Here's how the part is built. I have some questions about the finished solid (model axes, mm). A direction names the side the tool comes from. Round coordinates to 2 decimals unless told otherwise and drop trailing zeros. Write each loop counter-clockwise with the first axis right and the second up, starting at its lowest first coordinate (ties: lowest second). Pieces come first, ordered by that corner, then holes. Notation, with made-up numbers: (44.5, 47) - (101.5, 47) arc R28 ccw to (101.5, 73) - close; hole circle Ø7 at (37.5, 43). An arc over 180 degrees is marked (long way). Write item = value, one per line. Start each with the question number.
Item 1: If we section it at B-B (x = -73.5): Please give me the cut outline in (y, z).
Item 2: Which directions (+Z, -Z, +X, -X, +Y, -Y) give clear straight access to the entire face, cutting with the end or side of a thin tool? Please do faces 4 (the face through (6.37, 0.67, -105.56)), 5 (the face through (6, 54, -106.35)), 6 (the face through (2, 0, -1)).
Item 3: If we section it at A-A (y = 34): Please give me the cut outline in (x, z), and give its area (3 significant figures).
Item 4: If I drill on line 1 along Z through (x, y) = (10.5, 49.5); line 2 along Y through (x, z) = (47, -3.5); line 3 along X through (y, z) = (25, -90.5), over which ranges is the centre line in solid material (lowest first)? Write a range as [from, to].
Item 5: Thinking about a two-plate mould opening in Z: for faces 1 (the face through (-173.4, 54, -1)), 2 (the face through (1.58, 0.67, 105.56)), 3 (the face through (2, 54, 106.35)), which applies, pulls with the +Z half, pulls with the -Z half, needs draft (parallel to the pull), parting line crosses it, or undercut?
Item 6: If we section it at C-C (z = 25): Please give me the cut outline in (x, y).
Item 7: For P1, Ø6, axis at x = -53.5, z = 14, coming from the +Y side; P2, Ø8.5, axis at x = -171, y = 49.5, coming from the -Z side; P3, Ø6.5, axis at y = 34, z = 104.5, coming from the -X side; P4, Ø4, axis at x = -171.5, y = 37, coming from the +Z side, each with a flat end and sliding along its axis, tell me the tip position at first contact or that it passes through.
```python
from build123d import *

# Parameters (mm, degrees)
SKETCH1_W                    = 350
SKETCH1_H                    = 200
BASE_FLANGE1_DEPTH           = 1.6002
EDGE_FLANGE4_STRIP_W         = 19.1008
EDGE_FLANGE4_STRIP_H         = 1.6002
EDGE_FLANGE4_STRIP_CUT_DEPTH = 200
EDGE_FLANGE4_DEPTH           = 200
EDGE_FLANGE5_DEPTH           = 342.0498
EDGE_FLANGE5_BEND_DEPTH      = 342.0498


# Sheet-metal steps are written as plain solids
with BuildPart() as part:
    # Sketch1 → Base-Flange1 (new body)
    with BuildSketch(Plane(origin=(0, 0, 0), x_dir=(1, 0, 0), z_dir=(0, 1, 0))):
        Rectangle(SKETCH1_W, SKETCH1_H)
    extrude(amount=-BASE_FLANGE1_DEPTH)

    # Edge-Flange4 strip (across the edge) → Edge-Flange4 strip cut (cut)
    with BuildSketch(Plane(origin=(-175, 0, -100), x_dir=(1, 0, 0), z_dir=(0, 0, 1))):
        with Locations((-1.6002, -0.8001)):
            Rectangle(EDGE_FLANGE4_STRIP_W, EDGE_FLANGE4_STRIP_H)
    extrude(amount=EDGE_FLANGE4_STRIP_CUT_DEPTH, mode=Mode.SUBTRACT)

    # Edge-Flange4 section (across the edge) → Edge-Flange4 (add)
    with BuildSketch(Plane(origin=(-175, 0, -100), x_dir=(1, 0, 0), z_dir=(0, 0, 1))):
        with BuildLine():
            Line((0, 6.35), (0, 100))
            Line((0, 100), (1.6002, 100))
            Line((1.6002, 100), (1.6002, 6.35))
            ThreePointArc((1.6002, 6.35), (3.460071939, 1.859871939), (7.9502, 0))
            Line((7.9502, 0), (7.9502, -1.6002))
            ThreePointArc((7.9502, -1.6002), (2.328559668, 0.728359668), (0, 6.35))
        make_face()
    extrude(amount=EDGE_FLANGE4_DEPTH)

    # Edge-Flange5 section (across the edge) → Edge-Flange5 (add)
    with BuildSketch(Plane(origin=(-167.0498, 0, 106.35), x_dir=(0, 0, -1), z_dir=(1, 0, 0))):
        with BuildLine():
            Line((-1.6002, 6.35), (-1.6002, 100))
            Line((-1.6002, 100), (0, 100))
            Line((0, 100), (0, 6.35))
            ThreePointArc((0, 6.35), (1.859871939, 1.859871939), (6.35, 0))
            Line((6.35, 0), (6.35, -1.6002))
            ThreePointArc((6.35, -1.6002), (0.728359668, 0.728359668), (-1.6002, 6.35))
        make_face()
    extrude(amount=EDGE_FLANGE5_DEPTH)

    # Edge-Flange5 section 2 (across the edge) → Edge-Flange5 bend (add)
    with BuildSketch(Plane(origin=(175, 0, -106.35), x_dir=(0, 0, 1), z_dir=(-1, 0, 0))):
        with BuildLine():
            Line((-1.6002, 6.35), (-1.6002, 100))
            Line((-1.6002, 100), (0, 100))
            Line((0, 100), (0, 6.35))
            ThreePointArc((0, 6.35), (1.859871939, 1.859871939), (6.35, 0))
            Line((6.35, 0), (6.35, -1.6002))
            ThreePointArc((6.35, -1.6002), (0.728359668, 0.728359668), (-1.6002, 6.35))
        make_face()
    extrude(amount=EDGE_FLANGE5_BEND_DEPTH)


solid = part.part
```
Reply:
q1.outline = (-1.6, -100) arc R7.95 ccw to (6.35, -107.95) - (100, -107.95) - (100, -106.35) - (6.35, -106.35) arc R6.35 cw to (0, -100) - (0, 100) arc R6.35 cw to (6.35, 106.35) - (100, 106.35) - (100, 107.95) - (6.35, 107.95) arc R7.95 ccw to (-1.6, 100) - close
q2.face_4 = -Z, +X, -X, -Y
q2.face_5 = +X, -X, +Y
q2.face_6 = +X, +Y
q3.outline = (-175, -100) - (-173.4, -100) - (-173.4, 100) - (-175, 100) - close; (-167.05, -107.95) - (175, -107.95) - (175, -106.35) - (-167.05, -106.35) - close; (-167.05, 106.35) - (175, 106.35) - (175, 107.95) - (-167.05, 107.95) - close
q3.area = 1,410 mm2
q4.line_1 = [-107.95, -106.35], [106.35, 107.95]
q4.line_2 = [-1.6, 0]
q4.line_3 = [-175, -173.4]
q5.face_1 = needs draft
q5.face_2 = pulls with the +Z half
q5.face_3 = undercut
q6.outline = (-175, 6.35) arc R7.95 ccw to (-167.05, -1.6) - (175, -1.6) - (175, 0) - (-167.05, 0) arc R6.35 cw to (-173.4, 6.35) - (-173.4, 100) - (-175, 100) - close
q7.P1 = 0
q7.P2 = -107.95
q7.P3 = -167.05
q7.P4 = 100
